For this review, take the finished solid that the model builds, in its own axes (mm). Face numbers are marked on the shaded views. A direction names the side the tool comes from. Give positions to 0.01 mm unless a question says otherwise; leave off trailing zeros. Order: outer loops, then holes, each group sorted by start corner. A loop starts at its lowest first (then second) coordinate and runs counter-clockwise, first axis right, second up. Notation, with made-up numbers: (15, -40) - (50, -40) arc R14 cw to (50, -28) - close; hole circle Ø6 at (-30, 42). An arc over 180 degrees is marked (long way). Answer as a JSON object with one key per item and string values. Group by question number.
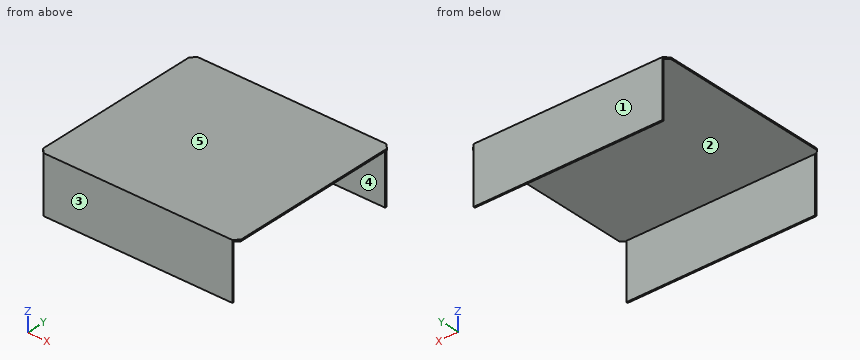
from build123d import *

# Parameters (mm, degrees)
F_5052_START                            = 86
F_5052_SHEET_TOP_PANEL_DEPTH            = 1.6
FOLDED_START                            = 27
SKETCH2_W                               = 202
SKETCH2_H                               = 1.6
FOLDED_SIDE_SKIRTS_WITH_OPEN_ENDS_DEPTH = 59


with BuildPart() as part:
    # Sketch1 → 5052 sheet top panel (new body)
    with BuildSketch(Plane.XY.offset(F_5052_START)):
        Polygon((-101, -96), (101, -96), (106, -91), (106, 91), (101, 96), (-101, 96), (-106, 91), (-106, -91), align=None)
    extrude(amount=F_5052_SHEET_TOP_PANEL_DEPTH)

    # Sketch2 → Folded side skirts with open ends (add)
    with BuildSketch(Plane.XY.offset(FOLDED_START)):
        with Locations((0, 95.2)):
            Rectangle(SKETCH2_W, SKETCH2_H)
        with Locations((0, -95.2)):
            Rectangle(SKETCH2_W, SKETCH2_H)
    extrude(amount=FOLDED_SIDE_SKIRTS_WITH_OPEN_ENDS_DEPTH)


solid = part.part
1) Consider section A-A (z = 41.5). Give the boundary of the cut face in (x, y).
2) For the marked faces 4 and 5, list the 3-axis set-ups (+Z, -Z, +X, -X, +Y, -Y) from which the entire face can be reached by the end or side of a thin tool; tool diameter is ignored.
3) Consider section B-B (x = -23.5). Give the boundary of the cut face in (y, z).
4) Consider section C-C (y = -36.5). Give the boundary of the cut face in (x, z), plus the area to 3 significant figures.
5) Mouldability with a two-part tool opening along Y and no side actions: class the marked faces 1, 2 and 3 as released by +Y, released by -Y, zero draft, split by the parting line, or undercut.
6) For pin 1 (1 mm diameter, centred on x = 69, y = -18.5, fed in from -Z); pin 2 (1.8 mm diameter, centred on y = -95, z = 49, fed in from -X); pin 3 (1.3 mm diameter, centred on y = -95, z = 70, fed in from +X), all flat-tipped, find the tip position at first contact; note any pin that passes through.
7) For line 1 (Y direction, x = 4, z = 69); line 2 (Z direction, x = -77, y = -48), list the stretches that pass through material, from the lowest coordinate up.
Result set:
{
 "1": {"outline": "(-101, -96) - (101, -96) - (101, -94.4) - (-101, -94.4) - close; (-101, 94.4) - (101, 94.4) - (101, 96) - (-101, 96) - close"},
 "2": {"face 4": "-Z, +X, -X", "face 5": "+Z, +X, -X, +Y, -Y"},
 "3": {"outline": "(-96, 27) - (-94.4, 27) - (-94.4, 86) - (94.4, 86) - (94.4, 27) - (96, 27) - (96, 87.6) - (-96, 87.6) - close"},
 "4": {"outline": "(-106, 86) - (106, 86) - (106, 87.6) - (-106, 87.6) - close", "area": "339 mm2"},
 "5": {"face 1": "released by +Y", "face 2": "undercut", "face 3": "released by -Y"},
 "6": {"pin 1": "stops at z = 86", "pin 2": "stops at x = -101", "pin 3": "stops at x = 101"},
 "7": {"line 1": "y = -96 to -94.4, 94.4 to 96", "line 2": "z = 86 to 87.6"}
}
